The figure shows three views and two pictorial views of one solid part (mm, origin at its lowest corner). Answer the questions. Coordinates: 2 decimals unless noted, no trailing zeros. Write each loop counter-clockwise with the first axis right and the second up, starting at its lowest first coordinate (ties: lowest second). Pieces come first, ordered by that corner, then holes.
Item 1: Straight lines are drawn through the part: probe 1 along Z at (x, y) = (19.05, 2.5); probe 2 along X at (y, z) = (5.5, 17.5). For each, find the intervals that lie inside material, in ascending order.
Item 2: Each of these flat-tipped pins is pushed along its axis until it touches: P1, Ø3, axis at y = 6, z = 41, coming from the -X side; P2, Ø4.5, axis at x = 19.05, z = 67.056, coming from the +Y side (3 decimals). Where does it stop, or does it pass through?
Item 3: Section A-A (x = 69.85) is taken. Give the vertices of the cut face in (y, z).
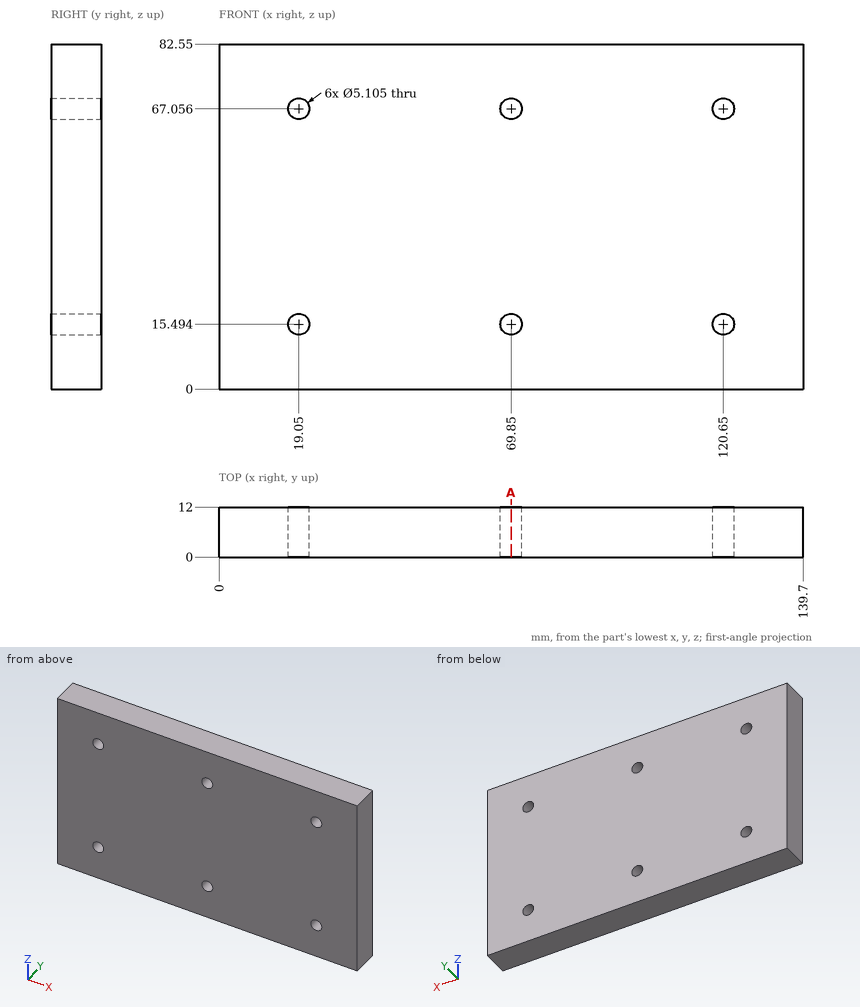
Established:
1. probe 1: z = 0 to 12.94, 18.05 to 64.5, 69.61 to 82.55
1. probe 2: x = 0 to 17.47, 20.63 to 68.27, 71.43 to 119.07, 122.23 to 139.7
2. P1: stops at x = 0
2. P2: passes through
3. outline: (0, 0) - (12, 0) - (12, 12.94) - (0, 12.94) - close; (0, 18.05) - (12, 18.05) - (12, 64.5) - (0, 64.5) - close; (0, 69.61) - (12, 69.61) - (12, 82.55) - (0, 82.55) - close
